```python
from build123d import *

# Parameters (mm, degrees)
CONECUT_DEPTH      = 27.521877713
CONECUT_DEPTH_BACK = 27.521877713


with BuildPart() as part:
    # Body: sweep along a path in 草图2
    with BuildLine(Plane.XY) as body_path:
        Line((22, 2.5), (0, 2.5))
        ThreePointArc((0, 2.5), (-1.229728386, 2.730698436), (-2.292225201, 3.391420912))
        ThreePointArc((-2.292225201, 3.391420912), (-10, 0), (-2.292225201, -3.391420912))
        ThreePointArc((-2.292225201, -3.391420912), (-1.229728386, -2.730698436), (0, -2.5))
        Line((0, -2.5), (26, -2.5))
    # 草图1 → Body (sweep)
    with BuildSketch(Plane(origin=(22, 0, 0), x_dir=(0, 0, -1), z_dir=(1, 0, 0))):
        with BuildLine():
            Line((-2.4999992, 0.002), (2.4999992, 0.002))
            ThreePointArc((2.4999992, 0.002), (0, 2.5), (-2.4999992, 0.002))
        make_face()
    sweep(path=body_path.line)

    # 草图3 → ConeCut (cut, two sides: drawn at the far end of the back side and taken through both)
    with BuildSketch(Plane.XY.offset(-CONECUT_DEPTH_BACK)):
        Polygon((22, 1.251), (20.210475082, 2.51), (26.01, 2.51), (26.01, -2.51), (24.210475082, -2.51), (26, -1.251), (24.204873421, 0), (20.204873421, 0), align=None)
    extrude(amount=CONECUT_DEPTH + CONECUT_DEPTH_BACK, mode=Mode.SUBTRACT)


solid = part.part
```
Build history of the part. All positions in model axes, mm. A direction names the side the tool comes from. Coordinates: 2 decimals unless noted, no trailing zeros. One line per question, with ' | ' between items. Start each with the question number.
1. Tool access for faces 5 (the face through (25.297, -1.745, -0.03)), 6 (the face through (10.8, 2.5, 0.1)): list every direction of +Z, -Z, +X, -X, +Y, -Y with a clear straight run to the whole face (end or side of a thin tool).
2. Mould opens along X. For faces 1 (the face through (21.32, 1.73, -0.03)), 2 (the face through (-7.5, 0.1, 0)), 3 (the face through (13.2, -2.5, 0.1)), 4 (the face through (-2.107, 0.392, -0.035)) say: +X half, -X half, draft (parallel to the pull), parting line (faces both ways), or undercut.
3. Wall check: line 1 along Y through (x, z) = (-5.4, 0); line 2 along Y through (x, z) = (-5.4, 1); line 3 along Z through (x, y) = (9, -1). Give the ranges that are in metal, low to high. Write a range as [from, to].
4. Flat gauge pin, fed straight in: P1, Ø3, axis at x = 4, y = -3, coming from the +Z side. Where does the tip first touch, or does it go through?
The answers:
1) face 5: +Z, -Z, +X, -Y | face 6: +X, +Y
2) face 1: +X half | face 2: undercut | face 3: draft | face 4: undercut
3) line 1: y = [-4.6, -2.1], [2.1, 4.6] | line 2: y = [-4.39, -2.1], [2.1, 4.39] | line 3: z = [-2.29, 2.29]
4) P1: stops at z = 2
